```python
from build123d import *

# Parameters (mm, degrees)
F0_W     = 12
F0_H     = 4
F1_DEPTH = 20
F2_W     = 5
F2_H     = 10
F3_DEPTH = 10
F4_DEPTH = 20
F5_R     = 0.5
F6_W     = 10
F6_H     = 10
F7_DEPTH = 15


with BuildPart() as f1:
    # F0 (on Front) → F1 (new body)
    with BuildSketch(Plane.XZ):
        Polygon((2.1224494493, 11), (-17.8775505507, 11), (-17.8775505507, 6), (-5.8775505507, 6), (2.1224494493, 6), align=None)
        Polygon((2.1224494493, -24), (2.1224494493, 6), (-5.8775505507, 6), (-5.8775505507, 4), (-5.8775505507, 0), (-5.8775505507, -14), (-5.8775505507, -24), align=None)
        with Locations((-11.8775505507, 2)):
            Rectangle(F0_W, F0_H)
    extrude(amount=F1_DEPTH)

    # F2 (on face) → F3 (join)
    with BuildSketch(Plane(origin=(-5.8775505507, 0, 0), x_dir=(0, -1, 0), z_dir=(-1, 0, 0))):
        with Locations((10, -19)):
            Rectangle(F2_W, F2_H)
    extrude(amount=F3_DEPTH)

    # F4 (add): a face of the model
    f4_faces = [f1.faces().sort_by_distance(p)[0] for p in [
        (-7.8775505507, -10, 11),
    ]]
    extrude(f4_faces, amount=F4_DEPTH)

    # F5
    f5_edges = [f1.edges().sort_by_distance(p)[0] for p in [
        (2.122449, -20, 3.5),
        (2.122449, 0, 3.5),
        (-1.877551, -20, -24),
        (-1.877551, 0, -24),
        (-10.877551, -12.5, -14),
        (-10.877551, -7.5, -14),
        (-15.877551, -10, -14),
        (-15.877551, -10, -24),
        (-10.877551, -12.5, -24),
        (-10.877551, -7.5, -24),
        (-7.877551, -20, 31),
        (-17.877551, -10, 31),
        (-7.877551, 0, 31),
        (2.122449, -10, 31),
    ]]
    fillet(f5_edges, radius=F5_R)

    # F6 (on face) → F7 (cut)
    with BuildSketch(Plane.XY.offset(31)):
        with Locations((-8.1275505507, -10)):
            Rectangle(F6_W, F6_H)
    extrude(amount=-F7_DEPTH, mode=Mode.SUBTRACT)


solid = f1.part
```
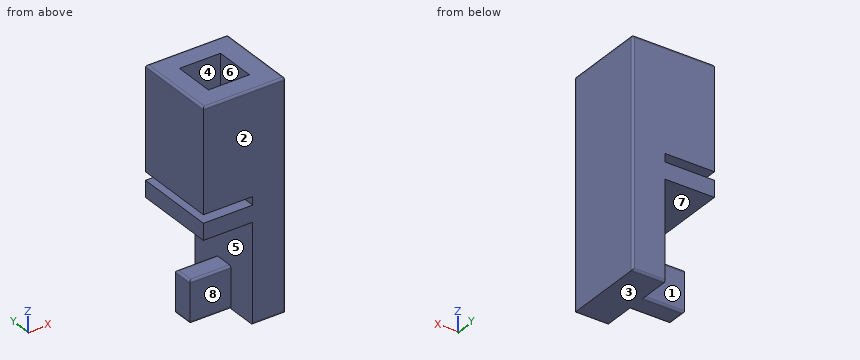
For this review, take the finished solid that the model builds, in its own axes (mm). Face numbers are marked on the shaded views. A direction names the side the tool comes from. Round coordinates to 2 decimals unless told otherwise and drop trailing zeros. Write each loop counter-clockwise with the first axis right and the second up, starting at its lowest first coordinate (ties: lowest second). Pieces come first, ordered by that corner, then holes.
1) Take a section at C-C on z = -18. Give the boundary of the cut face in (x, y), then the cut area to 3 significant figures.
Answer below:
outline: (-15.88, -12.5) - (-5.88, -12.5) - (-5.88, -20) - (1.62, -20) arc R0.5 ccw to (2.12, -19.5) - (2.12, -0.5) arc R0.5 ccw to (1.62, 0) - (-5.88, 0) - (-5.88, -7.5) - (-15.88, -7.5) - close
area: 210 mm2
2) Take a section at B-B on y = -4.25. Give the boundary of the cut face in (x, z).
Answer below:
outline: (-17.88, 0) - (-5.88, 0) - (-5.88, -24) - (2.12, -24) - (2.12, 30.5) arc R0.5 ccw to (1.62, 31) - (-17.38, 31) arc R0.5 ccw to (-17.88, 30.5) - (-17.88, 6) - (-5.88, 6) - (-5.88, 4) - (-17.88, 4) - close
3) Take a section at A-A on x = -13.75. Give the boundary of the cut face in (y, z), then the cut area to 3 significant figures.
Answer below:
outline: (-20, 0) - (0, 0) - (0, 4) - (-20, 4) - close; (-20, 6) - (0, 6) - (0, 30.5) arc R0.5 ccw to (-0.5, 31) - (-19.5, 31) arc R0.5 ccw to (-20, 30.5) - close; (-12.5, -23.5) arc R0.5 ccw to (-12, -24) - (-8, -24) arc R0.5 ccw to (-7.5, -23.5) - (-7.5, -14.5) arc R0.5 ccw to (-8, -14) - (-12, -14) arc R0.5 ccw to (-12.5, -14.5) - close
area: 630 mm2
4) Take a section at D-D on z = 27. Give the boundary of the cut face in (x, y).
Answer below:
outline: (-17.88, -20) - (1.62, -20) arc R0.5 ccw to (2.12, -19.5) - (2.12, -0.5) arc R0.5 ccw to (1.62, 0) - (-17.88, 0) - close; hole (-13.13, -15) - (-3.13, -15) - (-3.13, -5) - (-13.13, -5) - close
5) Insertion check: pin 1 Ø1.5 at (y, z) = (-10, -19) entering from -X; pin 2 Ø7 at (x, z) = (-12, -18.5) entering from +Y. Each pin has a flat end and moves straight along its axis. Give the tip position at first contact, or say it passes through.
Answer below:
pin 1: stops at x = -15.88
pin 2: stops at y = -7.5
6) Machinability: for the marked faces 5, 6, 7 and 8, which of the approach directions +Z, -Z, +X, -X, +Y, -Y give a long, thin tool a straight path to every point of the face, cutting with its end or side? Answer none if there is none.
Answer below:
face 5: -X
face 6: +Z
face 7: -X, +Y, -Y
face 8: -Z, -X, -Y
7) Mouldability with a two-part tool opening along Y and no side actions: class the marked faces 1, 2, 3 and 4 as +Y half, -Y half, draft (parallel to the pull), parting line (faces both ways), or undercut.
Answer below:
face 1: +Y half
face 2: -Y half
face 3: draft
face 4: undercut
8) For line 1 along Z through (x, y) = (-9.75, -14.5); line 2 along Z through (x, y) = (-6.5, -2.75); line 3 along Z through (x, y) = (-8.75, -8.75), list the stretches that pass through material, from the lowest coordinate up.
Answer below:
line 1: z = 0 to 4, 6 to 16
line 2: z = 0 to 4, 6 to 31
line 3: z = -24 to -14, 0 to 4, 6 to 16
